For this review, take the finished solid that the model builds, in its own axes (mm). Face numbers are marked on the shaded views. Round coordinates to 2 decimals unless told otherwise and drop trailing zeros. Order: outer loops, then holes, each group sorted by start corner. A loop starts at its lowest first (then second) coordinate and runs counter-clockwise, first axis right, second up. Notation, with made-up numbers: (85.25, 63) - (118.25, 63) arc R19 ccw to (118.25, 84) - close; hole circle Ø2 at (64.25, 60). An arc over 180 degrees is marked (long way). Write each question's results on one line, items separated by ' | '. Start each with the question number.
(1) Insertion check: pin 1 Ø17.5 at (x, z) = (10.5, 23.5) entering from -Y; pin 2 Ø0.5 at (y, z) = (22.5, -33) entering from +X (3 decimals); pin 3 Ø0.5 at (y, z) = (14.5, -32.5) entering from -X (3 decimals); pin 4 Ø6.5 at (y, z) = (7.62, 30.08) entering from -X. Each pin has a flat end and moves straight along its axis. Give the tip position at first contact, or say it passes through.
(2) Take a section at B-B, the plane x = 16. Give the boundary of the cut face in (y, z) (1 decimal), plus the area to 3 significant figures.
(3) For L1, parallel to X at y = 21.5, z = 29; L2, parallel to Z at x = 9, y = 50.5; L3, parallel to Y at x = 15, z = -17.5, list the stretches that pass through material, from the lowest coordinate up. Write a range as from..to.
(4) Take a section at A-A, the plane y = 7.62. Give the number of separate pieces and of enclosed holes in the cut face, plus the area to 3 significant figures.
(5) Take a section at C-C, the plane y = 52. Give the boundary of the cut face in (x, z), plus the area to 3 significant figures.
(6) Draft analysis for pull direction X (two halves, no side actions). For the marked faces 1, 2, 3 and 4, state which applies: pulls with the +X half, pulls with the -X half, needs draft (parallel to the pull), parting line crosses it, or undercut.
(7) Take a section at D-D, the plane z = -5. Give the boundary of the cut face in (x, y) (1 decimal), plus the area to 3 significant figures.
```python
from build123d import *

# Parameters (mm, degrees)
SKETCH1_W              = 65.94348
SKETCH1_H              = 76.02728
BOSS_EXTRUDE1_DEPTH    = 64.0969
CONVERT_SOLID1_START   = -29.75864
CONVERT_SOLID1_DEPTH   = 72.53478
CONVERT_SOLID1_START_2 = -34
CONVERT_SOLID1_2_DEPTH = 4.479485
CONVERT_SOLID1_START_3 = -32.01924
CONVERT_SOLID1_3_DEPTH = 64.03848
CONVERT_SOLID1_4_DEPTH = 1.98076
CONVERT_SOLID1_START_4 = 32.01924
CONVERT_SOLID1_5_DEPTH = 1.98076
CONVERT_SOLID1_START_5 = -32.97174
CONVERT_SOLID1_6_DEPTH = 3.730625
CONVERT_SOLID1_START_6 = 29.241115
CONVERT_SOLID1_7_DEPTH = 3.730625
CONVERT_SOLID1_START_7 = -29.520515
CONVERT_SOLID1_8_DEPTH = 73.520515
CUT_EXTRUDE4_REACH     = 106.765
SKETCH12_R             = 3.96875
CUT_EXTRUDE5_DEPTH     = 102.423632835


with BuildPart() as part:
    # Sketch1 → Boss-Extrude1 (new body)
    with BuildSketch(Plane(origin=(0, 0, 0), x_dir=(1, 0, 0), z_dir=(0, 1, 0))):
        with Locations((0, -4.7625)):
            Rectangle(SKETCH1_W, SKETCH1_H)
    extrude(amount=BOSS_EXTRUDE1_DEPTH)

    # Convert-Solid1: read off the stored shape, not the designer's step
    # Convert-Solid1 outline → Convert-Solid1 (cut)
    with BuildSketch(Plane.XY.offset(CONVERT_SOLID1_START)):
        with BuildLine():
            Line((-32.01924, 0), (32.01924, 0))
            Line((32.01924, 0), (32.01924, 60.6044))
            ThreePointArc((32.01924, 60.6044), (31.275291224, 62.400451224), (29.47924, 63.1444))
            Line((29.47924, 63.1444), (-29.47924, 63.1444))
            ThreePointArc((-29.47924, 63.1444), (-31.275291224, 62.400451224), (-32.01924, 60.6044))
            Line((-32.01924, 60.6044), (-32.01924, 0))
        make_face()
    extrude(amount=CONVERT_SOLID1_DEPTH, mode=Mode.SUBTRACT)

    # Convert-Solid1 2 outline → Convert-Solid1 2 (cut)
    with BuildSketch(Plane.XY.offset(CONVERT_SOLID1_START_2)):
        with BuildLine():
            Line((-30.605026438, 60.366275), (-29.241115, 60.366275))
            Line((-29.241115, 60.366275), (-29.241115, 63.1444))
            Line((-29.241115, 63.1444), (-29.47924, 63.1444))
            ThreePointArc((-29.47924, 63.1444), (-31.275291224, 62.400451224), (-32.01924, 60.6044))
            Line((-32.01924, 60.6044), (-32.01924, 0))
            Line((-32.01924, 0), (-30.605026438, 0))
            Line((-30.605026438, 0), (-30.605026438, 60.366275))
        make_face()
        with BuildLine():
            Line((29.47924, 63.1444), (29.241115, 63.1444))
            Line((29.241115, 63.1444), (29.241115, 60.366275))
            Line((29.241115, 60.366275), (30.605026438, 60.366275))
            Line((30.605026438, 60.366275), (30.605026438, 0))
            Line((30.605026438, 0), (32.01924, 0))
            Line((32.01924, 0), (32.01924, 60.6044))
            ThreePointArc((32.01924, 60.6044), (31.275291224, 62.400451224), (29.47924, 63.1444))
        make_face()
    extrude(amount=CONVERT_SOLID1_2_DEPTH, mode=Mode.SUBTRACT)

    # Convert-Solid1 3 outline → Convert-Solid1 3 (cut)
    with BuildSketch(Plane.YZ.offset(CONVERT_SOLID1_START_3)):
        with BuildLine():
            Line((63.1444, -29.75864), (63.1444, -29.520515))
            Line((63.1444, -29.520515), (60.366275, -29.520515))
            Line((60.366275, -29.520515), (60.366275, -29.75864))
            Line((60.366275, -29.75864), (0, -29.75864))
            Line((0, -29.75864), (0, -32.29864))
            Line((0, -32.29864), (60.6044, -32.29864))
            ThreePointArc((60.6044, -32.29864), (62.400451224, -31.554691224), (63.1444, -29.75864))
        make_face()
        with BuildLine():
            Line((64.0969, -33.25114), (64.0969, -29.75864))
            ThreePointArc((64.0969, -29.75864), (63.073970433, -32.228210433), (60.6044, -33.25114))
            Line((60.6044, -33.25114), (64.0969, -33.25114))
        make_face()
    extrude(amount=CONVERT_SOLID1_3_DEPTH, mode=Mode.SUBTRACT)

    # Convert-Solid1 4 outline → Convert-Solid1 4 (cut)
    with BuildSketch(Plane.YZ.offset(CONVERT_SOLID1_START_2)):
        Polygon((64.0969, 42.77614), (63.1444, 42.77614), (63.1444, -29.520515), (60.366275, -29.520515), (60.366275, -30.884426438), (0, -30.884426438), (0, -33.25114), (64.0969, -33.25114), align=None)
    extrude(amount=CONVERT_SOLID1_4_DEPTH, mode=Mode.SUBTRACT)

    # Convert-Solid1 5 outline → Convert-Solid1 5 (cut)
    with BuildSketch(Plane.YZ.offset(CONVERT_SOLID1_START_4)):
        Polygon((64.0969, 42.77614), (63.1444, 42.77614), (63.1444, -29.520515), (60.366275, -29.520515), (60.366275, -30.884426438), (0, -30.884426438), (0, -33.25114), (64.0969, -33.25114), align=None)
    extrude(amount=CONVERT_SOLID1_5_DEPTH, mode=Mode.SUBTRACT)

    # Convert-Solid1 6 outline → Convert-Solid1 6 (cut)
    with BuildSketch(Plane.YZ.offset(CONVERT_SOLID1_START_5)):
        with BuildLine():
            Line((64.0969, -29.75864), (64.0969, -29.520515))
            Line((64.0969, -29.520515), (63.1444, -29.520515))
            Line((63.1444, -29.520515), (63.1444, -29.75864))
            ThreePointArc((63.1444, -29.75864), (62.400451224, -31.554691224), (60.6044, -32.29864))
            Line((60.6044, -32.29864), (60.366275, -32.29864))
            Line((60.366275, -32.29864), (60.366275, -33.25114))
            Line((60.366275, -33.25114), (60.6044, -33.25114))
            ThreePointArc((60.6044, -33.25114), (63.073970433, -32.228210433), (64.0969, -29.75864))
        make_face()
    extrude(amount=CONVERT_SOLID1_6_DEPTH, mode=Mode.SUBTRACT)

    # Convert-Solid1 7 outline → Convert-Solid1 7 (cut)
    with BuildSketch(Plane.YZ.offset(CONVERT_SOLID1_START_6)):
        with BuildLine():
            Line((64.0969, -29.75864), (64.0969, -29.520515))
            Line((64.0969, -29.520515), (63.1444, -29.520515))
            Line((63.1444, -29.520515), (63.1444, -29.75864))
            ThreePointArc((63.1444, -29.75864), (62.400451224, -31.554691224), (60.6044, -32.29864))
            Line((60.6044, -32.29864), (60.366275, -32.29864))
            Line((60.366275, -32.29864), (60.366275, -33.25114))
            Line((60.366275, -33.25114), (60.6044, -33.25114))
            ThreePointArc((60.6044, -33.25114), (63.073970433, -32.228210433), (64.0969, -29.75864))
        make_face()
    extrude(amount=CONVERT_SOLID1_7_DEPTH, mode=Mode.SUBTRACT)

    # Convert-Solid1 8 outline → Convert-Solid1 8 (cut)
    with BuildSketch(Plane.XY.offset(CONVERT_SOLID1_START_7)):
        with BuildLine():
            Line((32.01924, 64.0969), (29.47924, 64.0969))
            ThreePointArc((29.47924, 64.0969), (31.948810433, 63.073970433), (32.97174, 60.6044))
            Line((32.97174, 60.6044), (32.97174, 63.1444))
            Line((32.97174, 63.1444), (32.01924, 63.1444))
            Line((32.01924, 63.1444), (32.01924, 64.0969))
        make_face()
        with BuildLine():
            ThreePointArc((-32.97174, 60.6044), (-31.948810433, 63.073970433), (-29.47924, 64.0969))
            Line((-29.47924, 64.0969), (-32.01924, 64.0969))
            Line((-32.01924, 64.0969), (-32.01924, 63.1444))
            Line((-32.01924, 63.1444), (-32.97174, 63.1444))
            Line((-32.97174, 63.1444), (-32.97174, 60.6044))
        make_face()
    extrude(amount=CONVERT_SOLID1_8_DEPTH, mode=Mode.SUBTRACT)

    # Sketch7 → Cut-Extrude4 (cut, up to next)
    with BuildSketch(Plane(origin=(0, 0, -33.25114), x_dir=(-1, 0, 0), z_dir=(0, 0, -1)), mode=Mode.PRIVATE) as cut_extrude4_sk1:
        with BuildLine():
            Line((-6.35, 23.1775), (-6.35, 0))
            Line((-6.35, 0), (6.35, 0))
            Line((6.35, 0), (6.35, 23.1775))
            ThreePointArc((6.35, 23.1775), (0, 29.5275), (-6.35, 23.1775))
        make_face()
    cut_extrude4_tool1 = extrude(cut_extrude4_sk1.sketch, amount=-CUT_EXTRUDE4_REACH, mode=Mode.PRIVATE) & part.part
    add(cut_extrude4_tool1.solids().sort_by_distance((0, 14.118049, -33.25114))[0], mode=Mode.SUBTRACT)

    # Sketch12 → Cut-Extrude5 (cut, through all)
    with BuildSketch(Plane.ZY.offset(32.97174)):
        with Locations((-18.184426438, 7.62)):
            Circle(SKETCH12_R)
        with Locations((30.07614, 7.62)):
            Circle(SKETCH12_R)
    extrude(amount=-CUT_EXTRUDE5_DEPTH, mode=Mode.SUBTRACT)


solid = part.part
```
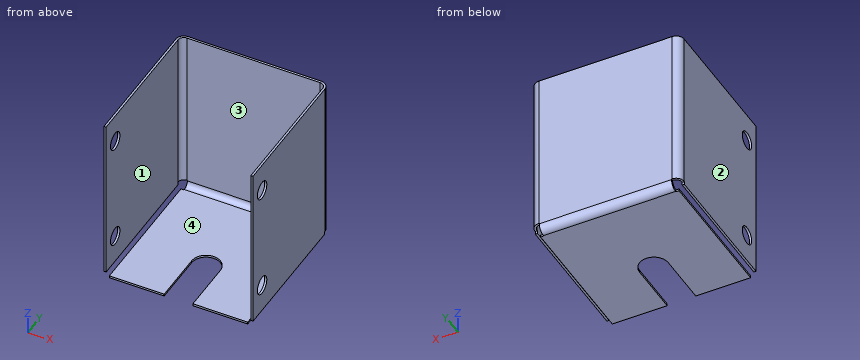
Results below:
1) pin 1: stops at y = 63.14 | pin 2: stops at x = 30.605 | pin 3: stops at x = -30.605 | pin 4: passes through
2) outline: (0, -33.3) - (60.6, -33.3) arc R3.5 ccw to (64.1, -29.8) - (64.1, 42.8) - (63.1, 42.8) - (63.1, -29.8) arc R2.5 cw to (60.6, -32.3) - (0, -32.3) - close | area: 131 mm^2
3) L1: x = -32.97..-32.02, 32.02..32.97 | L2: z = -33.25..-32.3 | L3: y = 63.14..64.1
4) separate pieces: 8 | enclosed holes: 0 | area: 156 mm^2
5) outline: (-32.97, -30.88) - (-32.02, -30.88) - (-32.02, 42.78) - (-32.97, 42.78) - close; (-30.61, -33.25) - (30.61, -33.25) - (30.61, -32.3) - (-30.61, -32.3) - close; (32.02, -30.88) - (32.97, -30.88) - (32.97, 42.78) - (32.02, 42.78) - close | area: 199 mm^2
6) face 1: undercut | face 2: pulls with the -X half | face 3: undercut | face 4: needs draft
7) outline: (-33, 0) - (-32, 0) - (-32, 60.6) arc R2.5 cw to (-29.5, 63.1) - (29.5, 63.1) arc R2.5 cw to (32, 60.6) - (32, 0) - (33, 0) - (33, 60.6) arc R3.5 ccw to (29.5, 64.1) - (-29.5, 64.1) arc R3.5 ccw to (-33, 60.6) - close | area: 181 mm^2
